The model under review builds one solid part; all positions refer to its coordinate system, in mm. Face numbers are marked on the shaded views. A direction names the side the tool comes from. Round coordinates to 2 decimals unless told otherwise and drop trailing zeros. Order: outer loops, then holes, each group sorted by start corner. A loop starts at its lowest first (then second) coordinate and runs counter-clockwise, first axis right, second up.
```python
from build123d import *

# Parameters (mm, degrees)
EXTRUDE_1_DEPTH     = 50
SKETCH_2_R          = 3.5
CUT_EXTRUDE_1_DEPTH = 98.247107926
SKETCH_3_R          = 1.95
EXTRUDE_2_DEPTH     = 5
CUT_EXTRUDE_2_REACH = 101.96
SKETCH_4_R          = 1.75
CHAMFER_1_SIZE      = 2
CHAMFER_2_SIZE      = 2
CHAMFER_3_SIZE      = 0.5
CUT_EXTRUDE_3_DEPTH = 2.5


with BuildPart() as part:
    # 草图1 → 凸台-拉伸1 (new, symmetric)
    with BuildSketch(Plane.XY):
        Polygon((-26, 45), (0, 45), (0, 49.079214745), (0, 51), (-60, 51), (-66, 51), (-66, 5), (-66, 0), (-55, 0), (-26, 0), align=None)
        Polygon((-31, 5), (-61, 5), (-61, 45), (-55, 45), (-31, 45), align=None, mode=Mode.SUBTRACT)
    extrude_1 = extrude(amount=EXTRUDE_1_DEPTH, both=True)

    # 镜向1: 凸台-拉伸1 across plane
    add(extrude_1.mirror(Plane(origin=(0, 0, 50), x_dir=(0, 0, 1), z_dir=(1, 0, 0))))

    # 草图2 → 切除-拉伸1 (cut, through all)
    with BuildSketch(Plane(origin=(0, 51, 0), x_dir=(1, 0, 0), z_dir=(0, 1, 0))):
        with Locations(Location((0, 0, 0), (0, 0, 270))):
            Circle(SKETCH_2_R)
    extrude(amount=-CUT_EXTRUDE_1_DEPTH, mode=Mode.SUBTRACT)

    # 草图3 → 凸台-拉伸2 (add)
    with BuildSketch(Plane(origin=(0, 51, 0), x_dir=(1, 0, 0), z_dir=(0, 1, 0))):
        with Locations(Location((44.45, 0, 0), (0, 0, 270))):
            Circle(SKETCH_3_R)
        with Locations(Location((-44.45, 0, 0), (0, 0, 90))):
            Circle(SKETCH_3_R)
    extrude(amount=EXTRUDE_2_DEPTH)

    # 草图4 → 切除-拉伸2 (cut, up to next)
    with BuildSketch(Plane.XZ, mode=Mode.PRIVATE) as cut_extrude_2_sk1:
        with Locations((-46, 35)):
            Circle(SKETCH_4_R)
    cut_extrude_2_tool1 = extrude(cut_extrude_2_sk1.sketch, amount=-CUT_EXTRUDE_2_REACH, mode=Mode.PRIVATE) & part.part
    # 草图4 → 切除-拉伸2 (cut, up to next)
    with BuildSketch(Plane.XZ, mode=Mode.PRIVATE) as cut_extrude_2_sk2:
        with Locations((46, 35)):
            Circle(SKETCH_4_R)
    cut_extrude_2_tool2 = extrude(cut_extrude_2_sk2.sketch, amount=-CUT_EXTRUDE_2_REACH, mode=Mode.PRIVATE) & part.part
    # 草图4 → 切除-拉伸2 (cut, up to next)
    with BuildSketch(Plane.XZ, mode=Mode.PRIVATE) as cut_extrude_2_sk3:
        with Locations((46, -35)):
            Circle(SKETCH_4_R)
    cut_extrude_2_tool3 = extrude(cut_extrude_2_sk3.sketch, amount=-CUT_EXTRUDE_2_REACH, mode=Mode.PRIVATE) & part.part
    # 草图4 → 切除-拉伸2 (cut, up to next)
    with BuildSketch(Plane.XZ, mode=Mode.PRIVATE) as cut_extrude_2_sk4:
        with Locations((-46, -35)):
            Circle(SKETCH_4_R)
    cut_extrude_2_tool4 = extrude(cut_extrude_2_sk4.sketch, amount=-CUT_EXTRUDE_2_REACH, mode=Mode.PRIVATE) & part.part
    add(cut_extrude_2_tool1.solids().sort_by_distance((-46, 0, 35))[0], mode=Mode.SUBTRACT)
    add(cut_extrude_2_tool2.solids().sort_by_distance((46, 0, 35))[0], mode=Mode.SUBTRACT)
    add(cut_extrude_2_tool3.solids().sort_by_distance((46, 0, -35))[0], mode=Mode.SUBTRACT)
    add(cut_extrude_2_tool4.solids().sort_by_distance((-46, 0, -35))[0], mode=Mode.SUBTRACT)

    # 倒角1
    chamfer_1_edges = [part.edges().sort_by_distance(p)[0] for p in [
        (-26, 45, 0),
        (26, 45, 0),
    ]]
    chamfer(chamfer_1_edges, length=CHAMFER_1_SIZE)

    # 倒角2
    chamfer_2_edges = [part.edges().sort_by_distance(p)[0] for p in [
        (0, 51, -50),
        (-66, 51, 0),
        (66, 51, 0),
        (0, 51, 50),
    ]]
    chamfer(chamfer_2_edges, length=CHAMFER_2_SIZE)

    # 倒角3
    chamfer_3_edges = [part.edges().sort_by_distance(p)[0] for p in [
        (0, 51, -3.5),
        (44.45, 56, -1.95),
        (-44.45, 56, 1.95),
    ]]
    chamfer(chamfer_3_edges, length=CHAMFER_3_SIZE)

    # 草图6 → 切除-拉伸3 (cut)
    with BuildSketch(Plane(origin=(0, 5, 0), x_dir=(1, 0, 0), z_dir=(0, 1, 0))):
        Polygon((42.535898385, 35), (44.267949192, 32), (47.732050808, 32), (49.464101615, 35), (47.732050808, 38), (44.267949192, 38), align=None)
        Polygon((-47.732050808, 32), (-44.267949192, 32), (-42.535898385, 35), (-44.267949192, 38), (-47.732050808, 38), (-49.464101615, 35), align=None)
        Polygon((-47.732050808, -38), (-44.267949192, -38), (-42.535898385, -35), (-44.267949192, -32), (-47.732050808, -32), (-49.464101615, -35), align=None)
        Polygon((42.535898385, -35), (44.267949192, -38), (47.732050808, -38), (49.464101615, -35), (47.732050808, -32), (44.267949192, -32), align=None)
    extrude(amount=-CUT_EXTRUDE_3_DEPTH, mode=Mode.SUBTRACT)


solid = part.part
```
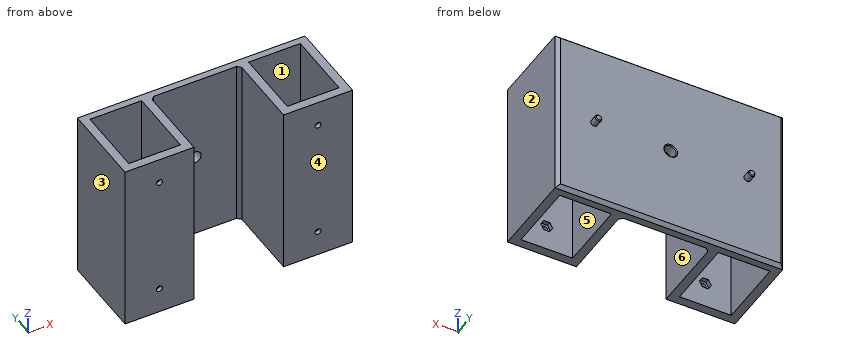
(1) Consider section D-D (z = 0). State how many separate pieces and enclosed holes the cut face has, and give its area (3 significant figures).
Data:
separate pieces: 2
enclosed holes: 2
area: 1,990 mm2
(2) Consider section C-C (z = -30). Write out the cut boundary in (x, y), and give its area (3 significant figures).
Data:
outline: (-66, 0) - (-26, 0) - (-26, 43) - (-24, 45) - (24, 45) - (26, 43) - (26, 0) - (66, 0) - (66, 49) - (64, 51) - (-64, 51) - (-66, 49) - close; hole (-61, 5) - (-31, 5) - (-31, 45) - (-61, 45) - close; hole (31, 5) - (61, 5) - (61, 45) - (31, 45) - close
area: 1,990 mm2
(3) Consider section B-B (y = 23.5). Write out the cut boundary in (x, z), and give its area (3 significant figures).
Data:
outline: (-66, -50) - (-61, -50) - (-61, 50) - (-66, 50) - close; (-31, -50) - (-26, -50) - (-26, 50) - (-31, 50) - close; (26, -50) - (31, -50) - (31, 50) - (26, 50) - close; (61, -50) - (66, -50) - (66, 50) - (61, 50) - close
area: 2,000 mm2
(4) To check wall thickness, follow probe 1 along X at (y, z) = (28, -15.5); probe 2 along Z at (x, y) = (-46, 1.4); probe 3 along Y at (x, z) = (35, 35.5). State the ranges of each line that lie inside material, in increasing order.
Data:
probe 1: x = -66 to -61, -31 to -26, 26 to 31, 61 to 66
probe 2: z = -50 to -36.75, -33.25 to 33.25, 36.75 to 50
probe 3: y = 0 to 5, 45 to 51
(5) For the marked faces 4, 5 and 6, list the 3-axis set-ups (+Z, -Z, +X, -X, +Y, -Y) from which the entire face can be reached by the end or side of a thin tool; tool diameter is ignored.
Data:
face 4: +Z, -Z, +X, -X, -Y
face 5: +Z, -Z
face 6: +Z, -Z, -Y
(6) Insertion check: pin 1 (6 mm diameter, centred on x = -9.5, z = 26.5, fed in from -Y); pin 2 (6.5 mm diameter, centred on x = -47, z = -34.5, fed in from +Y); pin 3 (6 mm diameter, centred on x = 45.5, y = 7.5, fed in from +Z). Each pin has a flat end and moves straight along its axis. Give the tip position at first contact, or say it passes through.
Data:
pin 1: stops at y = 45
pin 2: stops at y = 51
pin 3: stops at z = 50
(7) Consider section A-A (x = -35). Write out the cut boundary in (y, z), and give its area (3 significant figures).
Data:
outline: (0, -50) - (5, -50) - (5, 50) - (0, 50) - close; (45, -50) - (49, -50) - (51, -48) - (51, 48) - (49, 50) - (45, 50) - close
area: 1,100 mm2
(8) Draft analysis for pull direction X (two halves, no side actions). For the marked faces 1, 2 and 3, state which applies: pulls with the +X half, pulls with the -X half, needs draft (parallel to the pull), parting line crosses it, or undercut.
Data:
face 1: undercut
face 2: pulls with the +X half
face 3: pulls with the -X half
